from build123d import *

# Parameters (mm, degrees)
SKETCH1_W           = 45
SKETCH1_H           = 15
BOSS_EXTRUDE1_DEPTH = 5
BOSS_EXTRUDE2_DEPTH = 45
SKETCH5_R           = 8
CUT_EXTRUDE1_DEPTH  = 10
CUT_EXTRUDE2_REACH  = 39.075
SKETCH6_W           = 45
SKETCH6_H           = 8
SKETCH7_W           = 11
SKETCH7_H           = 10.717790556
CUT_EXTRUDE4_DEPTH  = 6.5
CUT_EXTRUDE5_REACH  = 39.075
SKETCH10_W          = 15
SKETCH10_H          = 16.318516526
BOSS_EXTRUDE3_DEPTH = 3
SKETCH11_W          = 15
SKETCH11_H          = 16.318516526
BOSS_EXTRUDE4_DEPTH = 3
SKETCH12_W          = 10
SKETCH12_H          = 7.679226714
CUT_EXTRUDE6_DEPTH  = 6
FILLET1_R           = 10
CUT_EXTRUDE7_DEPTH  = 0.5
CUT_EXTRUDE8_DEPTH  = 0.5


with BuildPart() as part:
    # Sketch1 → Boss-Extrude1 (new body)
    with BuildSketch(Plane(origin=(0, 0, 0), x_dir=(1, 0, 0), z_dir=(0, 1, 0))):
        with Locations((1.125, 2.045454545)):
            Rectangle(SKETCH1_W, SKETCH1_H)
    extrude(amount=BOSS_EXTRUDE1_DEPTH)

    # Sketch2 → Boss-Extrude2 (add)
    with BuildSketch(Plane(origin=(23.625, 0, 0), x_dir=(0, 0, -1), z_dir=(1, 0, 0))):
        Polygon((-2.454545455, 5), (2.721835448, 24.318516526), (-5.454545455, 24.318516526), (-5.454545455, 5), align=None)
        Polygon((1.168921177, 5), (6.345302079, 24.318516526), (9.545454545, 24.318516526), (9.545454545, 5), align=None)
    extrude(amount=-BOSS_EXTRUDE2_DEPTH)

    # Sketch5 → Cut-Extrude1 (cut)
    with BuildSketch(Plane(origin=(0, 0.948572854, 3.540122086), x_dir=(-1, 0, 0), z_dir=(0, -0.2588190451025247, -0.9659258262890673))):
        with Locations(Location((12.375, 14.194346021, 0), (0, 0, 90))):
            Circle(SKETCH5_R)
        with Locations(Location((-14.625, 14.194346021, 0), (0, 0, 90))):
            Circle(SKETCH5_R)
    extrude(amount=-CUT_EXTRUDE1_DEPTH, mode=Mode.SUBTRACT)

    # Cut-Extrude2: up to this plane
    cut_extrude2_end = Plane(origin=(-21.375, 5, 2.454545455), z_dir=(0, -0.2588190451025246, -0.9659258262890673))
    # Sketch6 → Cut-Extrude2 (cut, up to the surface)
    with BuildSketch(Plane.XY.offset(5.454545455), mode=Mode.PRIVATE) as cut_extrude2_sk1:
        with Locations((1.125, 20.318516526)):
            Rectangle(SKETCH6_W, SKETCH6_H)
    cut_extrude2_tool1 = split(extrude(cut_extrude2_sk1.sketch, amount=-CUT_EXTRUDE2_REACH, mode=Mode.PRIVATE), bisect_by=cut_extrude2_end, keep=Keep.BOTH, mode=Mode.PRIVATE)
    add(cut_extrude2_tool1.solids().sort_by_distance((1.125, 20.318517, 5.454545))[0], mode=Mode.SUBTRACT)

    # Sketch7 → Cut-Extrude4 (cut)
    with BuildSketch(Plane(origin=(0, 0.948572854, 3.540122086), x_dir=(-1, 0, 0), z_dir=(0, -0.2588190451025247, -0.9659258262890673))):
        with Locations((-1.125, 10.553241299)):
            Rectangle(SKETCH7_W, SKETCH7_H)
    extrude(amount=-CUT_EXTRUDE4_DEPTH, mode=Mode.SUBTRACT)


with BuildPart() as cut_extrude4_piece_1:
    # of the separate pieces the step leaves, piece 1, a body of its own (cut_extrude4_pieces)
    add(part.part.solids().sort_by_distance((-21.375, 0, -9.545454545))[0])


with BuildPart() as cut_extrude4_piece_2:
    # of the separate pieces the step leaves, piece 2, a body of its own (cut_extrude4_pieces)
    add(part.part.solids().sort_by_distance((-4.375, 16.318516526, -0.578241908))[0])


with BuildPart() as cut_extrude4_piece_3:
    # of the separate pieces the step leaves, piece 3, a body of its own (cut_extrude4_pieces)
    add(part.part.solids().sort_by_distance((6.811601533, 16.318516526, -0.578241908))[0])


with BuildPart() as cut_extrude5_tool:
    # Cut-Extrude5: up to this plane
    cut_extrude5_end = Plane(origin=(-21.375, 5, 2.454545455), z_dir=(0, -0.2588190451025246, -0.9659258262890673))
    # Sketch9 → Cut-Extrude5 (new, up to the surface)
    with BuildSketch(Plane.XY.offset(5.454545455), mode=Mode.PRIVATE) as cut_extrude5_sk1:
        Polygon((-12.375, 7.874399938), (-4.375, 6.839123758), (6.625, 6.839123758), (14.625, 7.874399938), (14.625, 17.142741254), (-12.375, 17.142741254), align=None)
    cut_extrude5_tool1 = split(extrude(cut_extrude5_sk1.sketch, amount=-CUT_EXTRUDE5_REACH, mode=Mode.PRIVATE), bisect_by=cut_extrude5_end, keep=Keep.BOTH, mode=Mode.PRIVATE)
    add(cut_extrude5_tool1.solids().sort_by_distance((1.125, 12.138424, 5.454545))[0])


with BuildPart() as cut_extrude4_piece_1_1:
    add(cut_extrude4_piece_1.part)

    # Cut-Extrude5: cut by cut_extrude5_tool
    add(cut_extrude5_tool.part, mode=Mode.SUBTRACT)

    # Sketch10 → Boss-Extrude3 (add)
    with BuildSketch(Plane.ZY.offset(21.375)):
        with Locations((-2.045454545, 8.159258263)):
            Rectangle(SKETCH10_W, SKETCH10_H)
    extrude(amount=BOSS_EXTRUDE3_DEPTH)

    # Sketch11 → Boss-Extrude4 (add)
    with BuildSketch(Plane(origin=(23.625, 0, 0), x_dir=(0, 0, -1), z_dir=(1, 0, 0))):
        with Locations((2.045454545, 8.159258263)):
            Rectangle(SKETCH11_W, SKETCH11_H)
    extrude(amount=BOSS_EXTRUDE4_DEPTH)

    # Sketch12 → Cut-Extrude6 (cut)
    with BuildSketch(Plane(origin=(0, 0.042706196, 0.159381694), x_dir=(1, 0, 0), z_dir=(0, 0.2588190451025247, 0.9659258262890673))):
        with Locations((1.125, 25.971781551)):
            Rectangle(SKETCH12_W, SKETCH12_H)
    extrude(amount=-CUT_EXTRUDE6_DEPTH, mode=Mode.SUBTRACT)

    # Fillet1
    # the kernel refuses this fillet: 10 mm, written as the material it adds along each edge
    with BuildSketch(Plane(origin=(-21.375, 16.318516526, 13.651862532), x_dir=(-1, 0, 0), z_dir=(0, 0, -1))) as fillet1_piece_1_section:
        with BuildLine():
            CenterArc((10, 7.141428429), FILLET1_R, 180, 45.572995999)
            Line((0, 7.141428429), (0, 0))
            Line((0, 0), (3, 0))
        make_face()
    fillet1_piece_1 = extrude(amount=23.197317077, mode=Mode.PRIVATE)
    fillet1_piece_1 = split(fillet1_piece_1, bisect_by=Plane(origin=(-22.137016454, 20.028758468, -5.195864872), z_dir=(0, -0.2588190451025247, -0.9659258262890673)), keep=Keep.TOP, mode=Mode.PRIVATE)
    add(fillet1_piece_1)
    with BuildSketch(Plane(origin=(23.625, 16.318516526, 13.651862532), x_dir=(1, 0, 0), z_dir=(0, 0, -1))) as fillet1_piece_2_section:
        with BuildLine():
            CenterArc((10, -7.141428429), FILLET1_R, 134.427004001, 45.572995999)
            Line((0, -7.141428429), (0, 0))
            Line((0, 0), (3, 0))
        make_face()
    fillet1_piece_2 = extrude(amount=23.197317077, mode=Mode.PRIVATE)
    fillet1_piece_2 = split(fillet1_piece_2, bisect_by=Plane(origin=(24.387016454, 20.028758468, -5.195864872), z_dir=(0, -0.2588190451025247, -0.9659258262890673)), keep=Keep.TOP, mode=Mode.PRIVATE)
    add(fillet1_piece_2)

    # Sketch14 → Cut-Extrude7 (cut)
    with BuildSketch(Plane(origin=(-21.375, 0, 0), x_dir=(0, 0, -1), z_dir=(1, 0, 0))):
        Polygon((0.578241908, 16.318516526), (4.201708539, 16.318516526), (1.168921177, 5), (-2.454545455, 5), align=None)
    extrude(amount=-CUT_EXTRUDE7_DEPTH, mode=Mode.SUBTRACT)

    # Sketch15 → Cut-Extrude8 (cut)
    with BuildSketch(Plane.ZY.offset(-23.625)):
        Polygon((-4.201708539, 16.318516526), (-0.578241908, 16.318516526), (2.454545455, 5), (-1.168921177, 5), align=None)
    extrude(amount=-CUT_EXTRUDE8_DEPTH, mode=Mode.SUBTRACT)


with BuildPart() as cut_extrude4_piece_2_1:
    add(cut_extrude4_piece_2.part)

    # Cut-Extrude5: cut by cut_extrude5_tool
    add(cut_extrude5_tool.part, mode=Mode.SUBTRACT)


with BuildPart() as cut_extrude4_piece_3_1:
    add(cut_extrude4_piece_3.part)

    # Cut-Extrude5: cut by cut_extrude5_tool
    add(cut_extrude5_tool.part, mode=Mode.SUBTRACT)


solid = cut_extrude4_piece_1_1.part
Could you check a few things on this model? Use its own coordinates, in mm. A direction names the side the tool comes from. Coordinates: 2 decimals unless noted, no trailing zeros. Order: outer loops, then holes, each group sorted by start corner. A loop starts at its lowest first (then second) coordinate and runs counter-clockwise, first axis right, second up. Notation, with made-up numbers: (58, 40.25) - (96, 40.25) arc R13 ccw to (96, 65.25) - close; hole circle Ø6 at (62, 3). An arc over 180 degrees is marked (long way). Answer in a Markdown table with one row per item. Add a question column.
(1) If we section it at B-B, the plane z = -1.75: Please give me the cut outline in (x, y) (3 decimals), then the cut area to 3 significant figures.
(2) I need wall thicknesses on L1, parallel to X at y = 14.25, z = -0.5 (3 decimals); L2, parallel to Y at x = 9, z = -0.5; L3, parallel to Y at x = -21, z = 3.25. Which ranges of each line are inside material? Lowest first, please.
(3) On a 3-axis mill with a long thin cutter (end or side, diameter ignored), from which of +Z, -Z, +X, -X, +Y, -Y can I reach the whole of each face in a straight line? I mean faces 5 (the face through (-22, 16.319, 2)), 6 (the face through (1.202, 6.396, 3.802)), 7 (the face through (6.125, 22, -8)), 8 (the face through (-18.781, 10.606, 3.256)). Say none if no direction works.
(4) If we section it at A-A, the plane x = 3.5: Please give me the cut outline in (y, z), then the cut area to 3 significant figures.
(5) If we section it at D-D, the plane z = -8.5: Please give me the cut outline in (x, y) (3 decimals), then the cut area to 3 significant figures.
(6) Will these pins go through, and if not, where does the flat tip stop? pin 1 (1.2 mm diameter, centred on y = 22, z = -8, fed in from +X); pin 2 (0.7 mm diameter, centred on y = 24, z = -7.5, fed in from -X) (3 decimals); pin 3 (1.8 mm diameter, centred on x = 10.5, z = 1.5, fed in from +Y).
(7) If we section it at C-C, the plane z = -5: Please give me the cut outline in (x, y) (3 decimals), then the cut area to 3 significant figures.
(8) If we mould it in two halves opening along Z, with no side actions, what happens to faces 1 (the face through (-21.875, 11, -1)), 2 (the face through (1.055, 20.895, -7.529)), 3 (the face through (1, 5, 1)), 4 (the face through (-13, 24.319, -8))? For each: released by +Z, released by -Z, zero draft, split by the parting line, or undercut.
Results are:
| question | item | result |
|---|---|---|
| 1 | outline | (-24.375, 0) - (26.625, 0) - (26.625, 16.319) - (24.125, 16.319) - (24.125, 7.169) - (-21.875, 7.169) - (-21.875, 16.319) - (-24.375, 16.319) - close |
| 1 | area | 411 mm2 |
| 2 | L1 | x = -24.375 to -21.875, 24.125 to 26.625 |
| 2 | L2 | y = 0 to 5 |
| 2 | L3 | y = 0 to 16.32 |
| 3 | face 5 | +Z, +X, -X, +Y |
| 3 | face 6 | +Y |
| 3 | face 7 | -Z, +Y |
| 3 | face 8 | none |
| 4 | outline | (0, -9.55) - (20.36, -9.55) - (21.42, -5.57) - (5, -1.17) - (5, 2.45) - (5.97, 2.2) - (6.84, 5.45) - (0, 5.45) - close |
| 4 | area | 179 mm2 |
| 5 | outline | (-24.375, 0) - (26.625, 0) - (26.625, 16.319) arc R10 cw to (23.625, 23.46) - (23.625, 24.319) - (6.125, 24.319) - (6.125, 20.635) - (-3.875, 20.635) - (-3.875, 24.319) - (-21.375, 24.319) - (-21.375, 23.46) arc R10 cw to (-24.375, 16.319) - close |
| 5 | area | 1,170 mm2 |
| 6 | pin 1 | stops at x = 23.84 |
| 6 | pin 2 | stops at x = -21.375 |
| 6 | pin 3 | stops at y = 7.45 |
| 7 | outline | (-24.375, 0) - (26.625, 0) - (26.625, 16.319) arc R10 cw to (24.532, 19.298) - (-22.282, 19.298) arc R10 cw to (-24.375, 16.319) - close |
| 7 | area | 977 mm2 |
| 8 | face 1 | undercut |
| 8 | face 2 | released by -Z |
| 8 | face 3 | undercut |
| 8 | face 4 | zero draft |
